Check sheet for the modelled part. Datum: model origin and axes. Units: mm. Face numbers are marked on the shaded views. Round coordinates to 2 decimals unless told otherwise and drop trailing zeros. Order: outer loops, then holes, each group sorted by start corner. A loop starts at its lowest first (then second) coordinate and runs counter-clockwise, first axis right, second up. Notation, with made-up numbers: (-8.5, 9.25) -> (7.5, 9.25) arc R11 ccw to (7.5, 14.25) -> close; hole circle Ø8 at (-9.75, 61). An arc over 180 degrees is marked (long way). Use CSV: the item, a comma, the result in double quotes.
Autodesk Inventor part; units mm, degrees
ref_plane "YZ Plane" through (0, 0, 0) normal (1, 0, 0) x (0, 1, 0)
ref_plane "XZ Plane" through (0, 0, 0) normal (0, 1, 0) x (-1, 0, 0)
ref_plane "XY Plane" through (0, 0, 0) normal (0, 0, 1) x (1, 0, 0)
sketch "スケッチ1" plane through (0, 0, 0) normal (0, 0, 1) x (1, 0, 0)
  circle A0 centre (0, 0) radius 4.05
  circle A1 centre (0, 0) radius 6.05
  dimension "d0" = 8.1
  dimension "d1" = 2
extrude "押し出し1" add sketch "スケッチ1" against normal blind 8.1
sketch "スケッチ2" plane through (0, 0, -8.1) normal (0, 0, -1) x (-1, 0, 0)
  circle A0 centre (0, 0) radius 6.05
  circle A1 centre (0, 0) radius 6.05
  dimension "d13" = 0
extrude "押し出し2" add sketch "スケッチ2" along normal blind 9
sketch "スケッチ3" plane through (0, 0, 0) normal (0, 1, 0) x (-1, 0, 0)
  circle A0 centre (0, -12.6) radius 1.25
  line L0 (4.05, -8.1) -> (-4.05, -8.1)
  point P0 (0, 0)
  dimension "d6" = 2.5
  dimension "d7" = 4.5
extrude "押し出し3" cut sketch "スケッチ3" along normal through all both and the other way through all
fillet "フィレット1" radius 1 2 edges at (6.05, 0, -17.1) (-6.05, 0, 0)
properties part number "parent_ver."
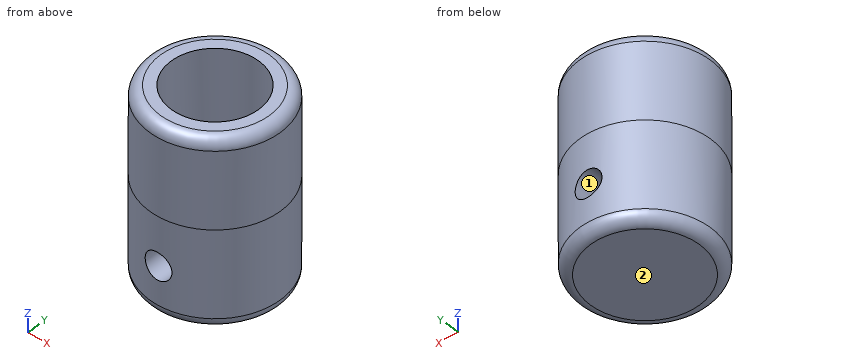
Q1. Mould release check, pull along X, two halves, no side actions. Record for the marked faces 1 and 2: pulls with the +X half, pulls with the -X half, needs draft (parallel to the pull), parting line crosses it, or undercut.
Result sheet:
face 1,"undercut"
face 2,"needs draft"
Q2. Sectioned sample at C-C, the plane z = -3.5. Enter the section's corners in (x, y), then the cut area to 3 significant figures.
Result sheet:
outline,"circle Ø12.1 at (0, 0); hole circle Ø8.1 at (0, 0)"
area,"63.5 mm^2"
Q3. Go/stop test with flat-tipped pins: pin 1 (3 mm diameter, centred on y = -4, z = -9.5, fed in from -X); pin 2 (2 mm diameter, centred on x = -4.5, z = -15, fed in from +Y); pin 3 (3 mm diameter, centred on y = 2.5, z = -13.5, fed in from +X). Record where each tip stops, or that it passes through.
Result sheet:
pin 1,"stops at x = -5.51"
pin 2,"stops at y = 4.93"
pin 3,"stops at x = 5.97"
Q4. Sectioned sample at A-A, the plane y = 0. Enter the section's corners in (x, z).
Result sheet:
outline,"(-6.05, -16.1) arc R1 ccw to (-5.05, -17.1) -> (5.05, -17.1) arc R1 ccw to (6.05, -16.1) -> (6.05, -1) arc R1 ccw to (5.05, 0) -> (4.05, 0) -> (4.05, -8.1) -> (-4.05, -8.1) -> (-4.05, 0) -> (-5.05, 0) arc R1 ccw to (-6.05, -1) -> close; hole circle Ø2.5 at (0, -12.6)"
Q5. Sectioned sample at B-B, the plane x = 0. Enter the section's corners in (y, z).
Result sheet:
outline,"(-6.05, -16.1) arc R1 ccw to (-5.05, -17.1) -> (5.05, -17.1) arc R1 ccw to (6.05, -16.1) -> (6.05, -13.85) -> (-6.05, -13.85) -> close; (-6.05, -11.35) -> (6.05, -11.35) -> (6.05, -1) arc R1 ccw to (5.05, 0) -> (4.05, 0) -> (4.05, -8.1) -> (-4.05, -8.1) -> (-4.05, 0) -> (-5.05, 0) arc R1 ccw to (-6.05, -1) -> close"
Q6. Scan lines: L1, parallel to Y at x = 0, z = -4.5; L2, parallel to Z at x = 0, y = 0.5; L3, parallel to Z at x = -3.25, y = -1.25. Record each from-to range of solid material in increasing order.
Result sheet:
L1,"y = -6.05 to -4.05, 4.05 to 6.05"
L2,"z = -17.1 to -13.85, -11.35 to -8.1"
L3,"z = -17.1 to -8.1"
Q7. Sectioned sample at D-D, the plane z = -12.6. Enter the section's corners in (x, y), then the cut area to 3 significant figures.
Result sheet:
outline,"(-1.25, -5.92) -> (-1.25, 5.92) arc R6.05 ccw to start; (1.25, -5.92) arc R6.05 ccw to (1.25, 5.92) -> close"
area,"85.0 mm^2"
